Could you check a few things on this model? Use its own coordinates, in mm. Face numbers are marked on the shaded views. A direction names the side the tool comes from. Give positions to 0.01 mm unless a question says otherwise; leave off trailing zeros. Loops run counter-clockwise (first coordinate to the right, second up) from the corner with the lowest first, then second, coordinate; pieces in that order, holes last. Notation, with made-up numbers: (52, 13.25) -> (83, 13.25) arc R30 cw to (83, 40.25) -> close; hole circle Ø7 at (-18.5, 37.25). An arc over 180 degrees is marked (long way). Put each result on its own line as item: value.
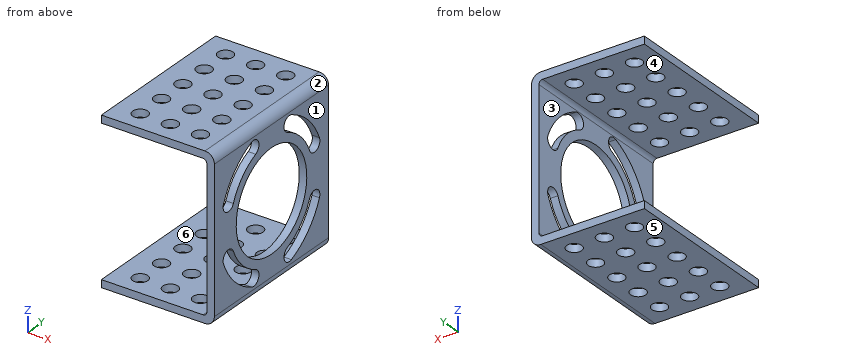
```python
from build123d import *

# Parameters (mm, degrees)
SKETCH1_W           = 42.9
SKETCH1_H           = 42.9
BOSS_EXTRUDE1_DEPTH = 2
SKETCH3_R           = 13.25
CUT_EXTRUDE2_DEPTH  = 61.702718226
SKETCH4_W           = 2
SKETCH4_H           = 42.9
BOSS_EXTRUDE2_DEPTH = 43
SKETCH5_R           = 2
SKETCH5_W           = 15
SKETCH5_H           = 42.9
CUT_EXTRUDE4_DEPTH  = 75.362759497
FILLET1_R           = 2.5
FILLET2_R           = 1


with BuildPart() as part:
    # Sketch1 → Boss-Extrude1 (new body)
    with BuildSketch(Plane(origin=(0, 0, 0), x_dir=(0, 0, -1), z_dir=(1, 0, 0))):
        with Locations((21.45, -21.45)):
            Rectangle(SKETCH1_W, SKETCH1_H)
    extrude(amount=BOSS_EXTRUDE1_DEPTH)

    # Sketch3 → Cut-Extrude2 (cut, through all)
    with BuildSketch(Plane.ZY):
        with Locations((-21.45, -21.45)):
            Circle(SKETCH3_R)
        with BuildLine():
            ThreePointArc((-39.465650884, -13.987673069), (-38.383258684, -16.600798999), (-35.770132754, -15.518406798))
            ThreePointArc((-35.770132754, -15.518406798), (-32.410155108, -10.489844892), (-27.381593202, -7.129867246))
            ThreePointArc((-27.381593202, -7.129867246), (-26.299201001, -4.516741316), (-28.912326931, -3.434349116))
            ThreePointArc((-28.912326931, -3.434349116), (-35.238582233, -7.661417767), (-39.465650884, -13.987673069))
        make_face()
        with BuildLine():
            ThreePointArc((-13.987673069, -3.434349116), (-16.600798999, -4.516741316), (-15.518406798, -7.129867246))
            ThreePointArc((-15.518406798, -7.129867246), (-10.489844892, -10.489844892), (-7.129867246, -15.518406798))
            ThreePointArc((-7.129867246, -15.518406798), (-4.516741316, -16.600798999), (-3.434349116, -13.987673069))
            ThreePointArc((-3.434349116, -13.987673069), (-7.661417767, -7.661417767), (-13.987673069, -3.434349116))
        make_face()
        with BuildLine():
            ThreePointArc((-3.434349116, -28.912326931), (-4.516741316, -26.299201001), (-7.129867246, -27.381593202))
            ThreePointArc((-7.129867246, -27.381593202), (-10.489844892, -32.410155108), (-15.518406798, -35.770132754))
            ThreePointArc((-15.518406798, -35.770132754), (-16.600798999, -38.383258684), (-13.987673069, -39.465650884))
            ThreePointArc((-13.987673069, -39.465650884), (-7.661417767, -35.238582233), (-3.434349116, -28.912326931))
        make_face()
        with BuildLine():
            ThreePointArc((-28.912326931, -39.465650884), (-26.299201001, -38.383258684), (-27.381593202, -35.770132754))
            ThreePointArc((-27.381593202, -35.770132754), (-32.410155108, -32.410155108), (-35.770132754, -27.381593202))
            ThreePointArc((-35.770132754, -27.381593202), (-38.383258684, -26.299201001), (-39.465650884, -28.912326931))
            ThreePointArc((-39.465650884, -28.912326931), (-35.238582233, -35.238582233), (-28.912326931, -39.465650884))
        make_face()
    extrude(amount=-CUT_EXTRUDE2_DEPTH, mode=Mode.SUBTRACT)

    # Sketch4 → Boss-Extrude2 (add)
    with BuildSketch(Plane.ZY):
        with Locations((-41.9, -21.45)):
            Rectangle(SKETCH4_W, SKETCH4_H)
        with Locations((-1, -21.45)):
            Rectangle(SKETCH4_W, SKETCH4_H)
    extrude(amount=BOSS_EXTRUDE2_DEPTH)

    # Sketch5 → Cut-Extrude4 (cut, through all)
    with BuildSketch(Plane(origin=(0, 0, -42.9), x_dir=(-1, 0, 0), z_dir=(0, 0, -1))):
        with Locations(Location((5.5, -5.487209302, 0), (0, 0, 90))):
            Circle(SKETCH5_R)
        with Locations(Location((13.5, -5.487209302, 0), (0, 0, 90))):
            Circle(SKETCH5_R)
        with Locations(Location((21.5, -5.487209302, 0), (0, 0, 90))):
            Circle(SKETCH5_R)
        with Locations(Location((13.5, -13.487209302, 0), (0, 0, 90))):
            Circle(SKETCH5_R)
        with Locations(Location((21.5, -13.487209302, 0), (0, 0, 90))):
            Circle(SKETCH5_R)
        with Locations(Location((13.5, -21.487209302, 0), (0, 0, 90))):
            Circle(SKETCH5_R)
        with Locations(Location((21.5, -21.487209302, 0), (0, 0, 90))):
            Circle(SKETCH5_R)
        with Locations(Location((13.5, -29.487209302, 0), (0, 0, 90))):
            Circle(SKETCH5_R)
        with Locations(Location((21.5, -29.487209302, 0), (0, 0, 90))):
            Circle(SKETCH5_R)
        with Locations(Location((13.5, -37.487209302, 0), (0, 0, 90))):
            Circle(SKETCH5_R)
        with Locations(Location((21.5, -37.487209302, 0), (0, 0, 90))):
            Circle(SKETCH5_R)
        with Locations(Location((5.5, -13.487209302, 0), (0, 0, 90))):
            Circle(SKETCH5_R)
        with Locations(Location((5.5, -21.487209302, 0), (0, 0, 90))):
            Circle(SKETCH5_R)
        with Locations(Location((5.5, -29.487209302, 0), (0, 0, 90))):
            Circle(SKETCH5_R)
        with Locations(Location((5.5, -37.487209302, 0), (0, 0, 90))):
            Circle(SKETCH5_R)
        with Locations((35.5, -21.45)):
            Rectangle(SKETCH5_W, SKETCH5_H)
    extrude(amount=-CUT_EXTRUDE4_DEPTH, mode=Mode.SUBTRACT)

    # Fillet1
    fillet1_edges = [part.edges().sort_by_distance(p)[0] for p in [
        (2, -21.45, -42.9),
        (2, -21.45, 0),
    ]]
    fillet(fillet1_edges, radius=FILLET1_R)

    # Fillet2
    fillet2_edges = [part.edges().sort_by_distance(p)[0] for p in [
        (0, -21.45, -40.9),
        (0, -21.45, -2),
    ]]
    fillet(fillet2_edges, radius=FILLET2_R)


solid = part.part
```
1. I'm going to push flat-ended pins straight in: pin 1 (6.5 mm diameter, centred on x = -5.5, y = -29.49, fed in from -Z); pin 2 (2 mm diameter, centred on y = -12, z = -37.5, fed in from -X). Where does each tip first touch, or does it pass through?
Recorded:
pin 1: stops at z = -42.9
pin 2: stops at x = 0
2. For the marked faces 5 and 6, which set-ups out of +Z, -Z, +X, -X, +Y, -Y let a thin tool reach every point of the face, with its end or its side?
Recorded:
face 5: -Z, +X, -X, +Y, -Y
face 6: -X, +Y, -Y
3. If we section it at B-B (x = -24.25): List the corners of the cut face in (y, z) for me, then the cut area to 3 significant figures.
Recorded:
outline: (-42.9, -42.9) -> (0, -42.9) -> (0, -40.9) -> (-42.9, -40.9) -> close; (-42.9, -2) -> (0, -2) -> (0, 0) -> (-42.9, 0) -> close
area: 172 mm^2
4. If we section it at C-C (z = -37): List the corners of the cut face in (x, y) for me, then the cut area to 3 significant figures.
Recorded:
outline: (0, -42.9) -> (2, -42.9) -> (2, -33.22) -> (0, -33.22) -> close; (0, -26.24) -> (2, -26.24) -> (2, -16.66) -> (0, -16.66) -> close; (0, -9.68) -> (2, -9.68) -> (2, 0) -> (0, 0) -> close
area: 57.9 mm^2
5. Thinking about a two-plate mould opening in Z: for the marked faces 1, 2, 3 and 4, which applies, pulls with the +Z half, pulls with the -Z half, needs draft (parallel to the pull), parting line crosses it, or undercut?
Recorded:
face 1: needs draft
face 2: pulls with the +Z half
face 3: undercut
face 4: undercut
6. If we section it at D-D (y = -34): List the corners of the cut face in (x, z) for me, then the cut area to 3 significant figures.
Recorded:
outline: (-28, -42.9) -> (-0.5, -42.9) arc R2.5 ccw to (2, -40.4) -> (2, -36.37) -> (0, -36.37) -> (0, -39.9) arc R1 cw to (-1, -40.9) -> (-28, -40.9) -> close; (-28, -2) -> (-1, -2) arc R1 cw to (0, -3) -> (0, -6.53) -> (2, -6.53) -> (2, -2.5) arc R2.5 ccw to (-0.5, 0) -> (-28, 0) -> close; (0, -30.55) -> (2, -30.55) -> (2, -25.7) -> (0, -25.7) -> close; (0, -17.2) -> (2, -17.2) -> (2, -12.35) -> (0, -12.35) -> close
area: 155 mm^2
7. If we section it at A-A (z = -21.45): List the corners of the cut face in (x, y) for me.
Recorded:
outline: (0, -42.9) -> (2, -42.9) -> (2, -34.7) -> (0, -34.7) -> close; (0, -8.2) -> (2, -8.2) -> (2, 0) -> (0, 0) -> close
8. I need wall thicknesses on line 1 (Z direction, x = -2, y = -36.5); line 2 (X direction, y = -8, z = -15). Which ranges of each line are inside material? Lowest first, please.
Recorded:
line 1: z = -42.9 to -40.9, -2 to 0
line 2: x = 0 to 2
